```python
from build123d import *

# Parameters (mm, degrees)
BOSS_EXTRUDE1_DEPTH   = 300
SKETCH2_R             = 1.75
CUT_EXTRUDE1_DEPTH    = 10
SKETCH3_R             = 3
CUT_EXTRUDE2_DEPTH    = 4
CHAMFER1_SIZE         = 0.5
CHAMFER1_SIZE2        = 1.743707222
CHAMFER1_PART_2_SIZE  = 0.5
CHAMFER1_PART_2_SIZE2 = 1.743707222
FILLET1_R             = 0.5


with BuildPart() as part:
    # Sketch1 → Boss-Extrude1 (new body)
    with BuildSketch(Plane(origin=(0, 0, 0), x_dir=(0, 0, -1), z_dir=(1, 0, 0))):
        Polygon((-0.5, 6), (4, 6), (4, -6), (-0.5, -6), (-0.5, -4.25), (-2.5, -4.25), (-2.5, -6), (-4, -6), (-4, 6), (-2.5, 6), (-2.5, 4.25), (-0.5, 4.25), align=None)
    extrude(amount=BOSS_EXTRUDE1_DEPTH)

    # Sketch2 → Cut-Extrude1 (cut)
    with BuildSketch(Plane.XY.offset(4)):
        with Locations((13, 0)):
            Circle(SKETCH2_R)
        with Locations((38, 0)):
            Circle(SKETCH2_R)
        with Locations((63, 0)):
            Circle(SKETCH2_R)
        with Locations((88, 0)):
            Circle(SKETCH2_R)
        with Locations((113, 0)):
            Circle(SKETCH2_R)
        with Locations((138, 0)):
            Circle(SKETCH2_R)
        with Locations((163, 0)):
            Circle(SKETCH2_R)
        with Locations((188, 0)):
            Circle(SKETCH2_R)
        with Locations((213, 0)):
            Circle(SKETCH2_R)
        with Locations((238, 0)):
            Circle(SKETCH2_R)
        with Locations((263, 0)):
            Circle(SKETCH2_R)
        with Locations((288, 0)):
            Circle(SKETCH2_R)
        with Locations((313, 0)):
            Circle(SKETCH2_R)
        with Locations((338, 0)):
            Circle(SKETCH2_R)
        with Locations((363, 0)):
            Circle(SKETCH2_R)
        with Locations((388, 0)):
            Circle(SKETCH2_R)
    extrude(amount=-CUT_EXTRUDE1_DEPTH, mode=Mode.SUBTRACT)

    # Sketch3 → Cut-Extrude2 (cut)
    with BuildSketch(Plane.XY.offset(4)):
        with Locations((13, 0)):
            Circle(SKETCH3_R)
        with Locations((38, 0)):
            Circle(SKETCH3_R)
        with Locations((63, 0)):
            Circle(SKETCH3_R)
        with Locations((88, 0)):
            Circle(SKETCH3_R)
        with Locations((113, 0)):
            Circle(SKETCH3_R)
        with Locations((138, 0)):
            Circle(SKETCH3_R)
        with Locations((163, 0)):
            Circle(SKETCH3_R)
        with Locations((188, 0)):
            Circle(SKETCH3_R)
        with Locations((213, 0)):
            Circle(SKETCH3_R)
        with Locations((238, 0)):
            Circle(SKETCH3_R)
        with Locations((263, 0)):
            Circle(SKETCH3_R)
        with Locations((288, 0)):
            Circle(SKETCH3_R)
        with Locations((313, 0)):
            Circle(SKETCH3_R)
        with Locations((338, 0)):
            Circle(SKETCH3_R)
        with Locations((363, 0)):
            Circle(SKETCH3_R)
        with Locations((388, 0)):
            Circle(SKETCH3_R)
    extrude(amount=-CUT_EXTRUDE2_DEPTH, mode=Mode.SUBTRACT)

    # Chamfer1
    chamfer1_edges = [part.edges().sort_by_distance(p)[0] for p in [
        (150, -4.25, 0.5),
        (150, -4.25, 2.5),
    ]]
    chamfer1_side = [part.faces().sort_by_distance(p)[0] for p in [
        (150, -4.25, 1.5),
    ]]
    chamfer(chamfer1_edges, length=CHAMFER1_SIZE, length2=CHAMFER1_SIZE2, reference=chamfer1_side[0])

    # Chamfer1 part 2
    chamfer1_part_2_edges = [part.edges().sort_by_distance(p)[0] for p in [
        (150, 4.25, 2.5),
        (150, 4.25, 0.5),
    ]]
    chamfer1_part_2_side = [part.faces().sort_by_distance(p)[0] for p in [
        (150, 4.25, 1.5),
    ]]
    chamfer(chamfer1_part_2_edges, length=CHAMFER1_PART_2_SIZE, length2=CHAMFER1_PART_2_SIZE2, reference=chamfer1_part_2_side[0])

    # Fillet1
    fillet1_edges = [part.edges().sort_by_distance(p)[0] for p in [
        (300, -6, -1.75),
        (300, 0, -4),
        (300, 6, -1.75),
        (300, 6, 3.25),
        (300, 0, 4),
        (300, -6, 3.25),
        (0, -6, 3.25),
        (0, -6, -1.75),
        (0, 0, -4),
        (0, 6, -1.75),
        (0, 6, 3.25),
        (0, 0, 4),
        (150, -4.25, 1),
        (150, -4.25, 2),
        (150, 4.25, 2),
        (150, 4.25, 1),
        (150, -6, 4),
        (150, 6, 4),
        (150, -6, -4),
        (150, 6, -4),
    ]]
    fillet(fillet1_edges, radius=FILLET1_R)


solid = part.part
```
Build history of the part. All positions in model axes, mm. Round coordinates to 2 decimals unless told otherwise and drop trailing zeros. Use a Markdown table: item, result.
1) Flat gauge pins, fed straight in: pin 1 Ø1.8 at (x, y) = (61.5, 0) entering from +Z; pin 2 Ø7 at (x, y) = (138, 0) entering from -Z; pin 3 Ø2 at (x, y) = (38, 0) entering from -Z. Where does each tip first touch, or does it go through?
Recorded:
| item | result |
|---|---|
| pin 1 | stops at z = 0 |
| pin 2 | stops at z = -4 |
| pin 3 | passes through |
2) Wall check: L1, parallel to Y at x = 113, z = -1.75; L2, parallel to Y at x = 188, z = 1.25; L3, parallel to Z at x = 219.5, y = 5. Give the ranges that are in metal, low to high.
Recorded:
| item | result |
|---|---|
| L1 | y = -6 to -1.75, 1.75 to 6 |
| L2 | y = -4.27 to -3, 3 to 4.27 |
| L3 | z = -4 to 0.78, 2.22 to 4 |
3) Saw through at B-B on z = -1.5. Give the number of separate pieces and of enclosed holes in the cut face, and give its area (3 significant figures).
Recorded:
| item | result |
|---|---|
| separate pieces | 1 |
| enclosed holes | 12 |
| area | 3,480 mm² |
4) Pull direction X, two halves, no side cores. Call faces 1 (the face through (300, 0, 0)), 2 (the face through (10, 0, 2)), 3 (the face through (148, 0, -4)), 4 (the face through (0, 0, 0)): pulls with the +X half, pulls with the -X half, needs draft (parallel to the pull), parting line crosses it, or undercut.
Recorded:
| item | result |
|---|---|
| face 1 | pulls with the +X half |
| face 2 | undercut |
| face 3 | needs draft |
| face 4 | pulls with the -X half |
